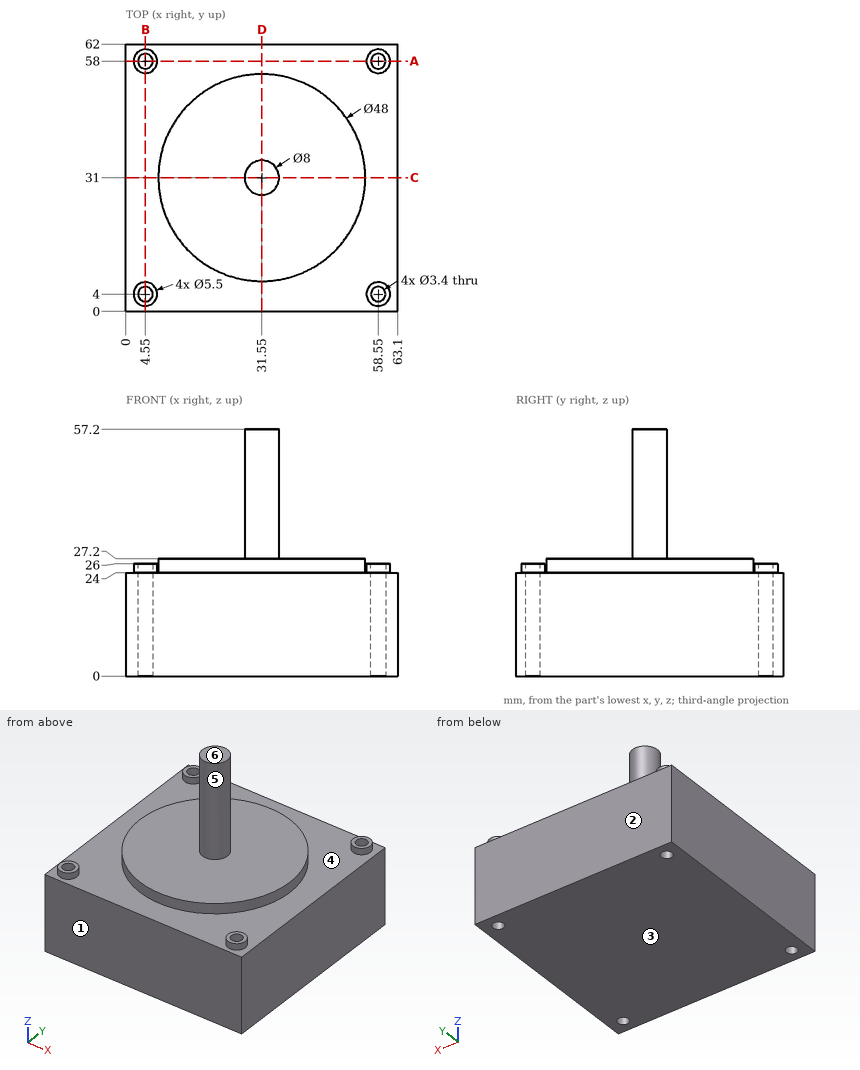
For this review, use the dimensioned drawing (mm, ordinates from the lowest corner) and the shaded views. A direction names the side the tool comes from. Coordinates: 2 decimals unless noted, no trailing zeros. Loops run counter-clockwise (first coordinate to the right, second up) from the corner with the lowest first, then second, coordinate; pieces in that order, holes last.
1. Mouldability with a two-part tool opening along Y and no side actions: class the marked faces 1, 2, 3 and 4 as +Y half, -Y half, draft (parallel to the pull), parting line (faces both ways), or undercut.
2. For line 1 (Y direction, x = 58.55, z = 12.75); line 2 (Y direction, x = 58, z = 6); line 3 (Y direction, x = 59, z = 25), list the stretches that pass through material, from the lowest coordinate up.
3. Add section D-D, the plane x = 31.55. Give the boundary of the cut face in (y, z), then the cut area to 3 significant figures.
4. Add section A-A, the plane y = 58. Give the boundary of the cut face in (x, z), then the cut area to 3 significant figures.
5. Insertion check: P1, Ø10, axis at y = 38, z = 51, coming from the +X side; P2, Ø3, axis at x = 59, y = 58, coming from the +Z side; P3, Ø18.5, axis at x = 23, y = 44, coming from the +Z side. Each pin has a flat end and moves straight along its axis. Give the tip position at first contact, or say it passes through.
6. For the marked faces 5 and 6, list the 3-axis set-ups (+Z, -Z, +X, -X, +Y, -Y) from which the entire face can be reached by the end or side of a thin tool; tool diameter is ignored.
7. Add section C-C, the plane y = 31. Give the boundary of the cut face in (x, z).
8. Add section B-B, the plane x = 4.55. Give the boundary of the cut face in (y, z).
Result:
1. face 1: -Y half
1. face 2: +Y half
1. face 3: draft
1. face 4: undercut
2. line 1: y = 0 to 2.3, 5.7 to 56.3, 59.7 to 62
2. line 2: y = 0 to 2.39, 5.61 to 56.39, 59.61 to 62
2. line 3: y = 1.29 to 2.36, 5.64 to 6.71, 55.29 to 56.36, 59.64 to 60.71
3. outline: (0, 0) - (62, 0) - (62, 24) - (55, 24) - (55, 27.2) - (35, 27.2) - (35, 57.2) - (27, 57.2) - (27, 27.2) - (7, 27.2) - (7, 24) - (0, 24) - close
3. area: 1,880 mm2
4. outline: (0, 0) - (2.85, 0) - (2.85, 26) - (1.8, 26) - (1.8, 24) - (0, 24) - close; (6.25, 0) - (56.85, 0) - (56.85, 26) - (55.8, 26) - (55.8, 24) - (7.3, 24) - (7.3, 26) - (6.25, 26) - close; (60.25, 0) - (63.1, 0) - (63.1, 24) - (61.3, 24) - (61.3, 26) - (60.25, 26) - close
4. area: 1,360 mm2
5. P1: stops at x = 35.01
5. P2: stops at z = 26
5. P3: stops at z = 27.2
6. face 5: +Z
6. face 6: +Z, +X, -X, +Y, -Y
7. outline: (0, 0) - (63.1, 0) - (63.1, 24) - (55.55, 24) - (55.55, 27.2) - (35.55, 27.2) - (35.55, 57.2) - (27.55, 57.2) - (27.55, 27.2) - (7.55, 27.2) - (7.55, 24) - (0, 24) - close
8. outline: (0, 0) - (2.3, 0) - (2.3, 26) - (1.25, 26) - (1.25, 24) - (0, 24) - close; (5.7, 0) - (56.3, 0) - (56.3, 26) - (55.25, 26) - (55.25, 24) - (6.75, 24) - (6.75, 26) - (5.7, 26) - close; (59.7, 0) - (62, 0) - (62, 24) - (60.75, 24) - (60.75, 26) - (59.7, 26) - close
